For this review, take the finished solid that the model builds, in its own axes (mm). A direction names the side the tool comes from. Give positions to 0.01 mm unless a question says otherwise; leave off trailing zeros. Write each loop counter-clockwise with the first axis right and the second up, starting at its lowest first coordinate (ties: lowest second). Pieces come first, ordered by that corner, then holes.
1) We need section B-B on y = 0. Give the boundary of the cut face in (x, z).
2) For P1, Ø2, axis at x = -11.5, y = 34, coming from the +Z side; P2, Ø1.6, axis at x = -24, z = 14.5, coming from the -Y side; P3, Ø22.5, axis at y = -1.5, z = 18, coming from the -X side, all flat-tipped, find the tip position at first contact; note any pin that passes through.
3) Draft analysis for pull direction X (two halves, no side actions). For faces 4 (the face through (-11.923, 53.692, 2.348)), 5 (the face through (-23.5, 0, 23)), 6 (the face through (-24.486, -0.11, 35.764)), 7 (the face through (-1, 1, 4.762)), state which applies: pulls with the +X half, pulls with the -X half, needs draft (parallel to the pull), parting line crosses it, or undercut.
4) Wall thickness on line 1 along X through (y, z) = (-3, 9.5); line 2 along Z through (x, y) = (6.5, -30.5); line 3 along Y through (x, z) = (-25, 35.5): over which ranges is each line inside the solid? List them lowest first.
5) We need section A-A on z = 16.5. Give the boundary of the cut face in (x, y), and give its area (3 significant figures).
6) Machinability: for faces 1 (the face through (23.5, 0, 23)), 2 (the face through (-25.5, 0, 23)), 3 (the face through (25.5, 0, 23)), which of the approach directions +Z, -Z, +X, -X, +Y, -Y give a long, thin tool a straight path to every point of the face, cutting with its end or side? Answer none if there is none.
7) We need section D-D on x = 0. Give the boundary of the cut face in (y, z).
8) We need section C-C on z = 38. Give the boundary of the cut face in (x, y), and give its area (3 significant figures).
Autodesk Inventor part; units mm, degrees
ref_plane "YZ Plane" through (0, 0, 0) normal (1, 0, 0) x (0, 1, 0)
ref_plane "XZ Plane" through (0, 0, 0) normal (0, 1, 0) x (-1, 0, 0)
ref_plane "XY Plane" through (0, 0, 0) normal (0, 0, 1) x (1, 0, 0)
sketch "Sketch1" plane through (0, 0, 0) normal (0, 0, 1) x (1, 0, 0)
  circle A0 centre (0, 0) radius 55
  line L0 (23.5, -14) -> (23.5, 14)
  line L1 (-23.5, -14) -> (-23.5, 14)
  line L2 (-25.5, -14) -> (-25.5, 14)
  line L3 (25.5, -14) -> (25.5, 14)
  line L4 (25.5, 14) -> (23.5, 14)
  line L5 (23.5, -14) -> (25.5, -14)
  line L6 (-25.5, -14) -> (-23.5, -14)
  line L7 (-25.5, 14) -> (-23.5, 14)
extrude "Extrusion1" add sketch "Sketch1" along normal blind 4.7625
extrude "Extrusion2" add sketch "Sketch1" along normal blind 40.7625 contours L0 L4 L3 L5 | L6 L2 L7 L1
sketch "Sketch2" plane through (25.5, -14, 4.7625) normal (1, 0, 0) x (0, 0, -1)
  line L0 (-36, 28) -> (-36, 0)
  line L1 (-39, 7) -> (-39, 2.0417)
  arc A0 (-39, 2.0417) -> (-37.1667, 0.0487) centre (-37, 2.0417) ccw
  arc A1 (-37.1667, 0.0487) -> (-36, 0) centre (-36, 14) ccw
  line L2 (-2, 0) -> (-36, 0)
  line L3 (-2, 28) -> (-2, 0)
  line L4 (-2, 28) -> (-36, 28)
  arc A2 (-36, 28) -> (-37.1667, 27.9513) centre (-36, 14) ccw
  arc A3 (-37.1667, 27.9513) -> (-39, 25.9583) centre (-37, 25.9583) ccw
  line L5 (-39, 25.9583) -> (-39, 21)
  arc A4 (-39, 21) -> (-37, 19) centre (-37, 21) ccw
  line L6 (-37, 19) -> (-36, 19)
  arc A5 (-36, 9) -> (-36, 19) centre (-36, 14) ccw
  line L7 (-37, 9) -> (-36, 9)
  arc A6 (-37, 9) -> (-39, 7) centre (-37, 7) ccw
  circle A7 centre (-36, 25) radius 1.25
  circle A8 centre (-28.2218, 21.7782) radius 1.25
  circle A9 centre (-25, 14) radius 1.25
  circle A10 centre (-28.2218, 6.2218) radius 1.25
  circle A11 centre (-36, 3) radius 1.25
  circle A12 centre (-15, 6) radius 1.05
  circle A13 centre (-15, 22) radius 1.05
  line L8 (-8, 6) -> (-11, 6)
  arc A14 (-12, 7) -> (-11, 6) centre (-11, 7) ccw
  line L9 (-12, 7) -> (-12, 21)
  arc A15 (-11, 22) -> (-12, 21) centre (-11, 21) ccw
  line L10 (-8, 22) -> (-11, 22)
  arc A16 (-7, 21) -> (-8, 22) centre (-8, 21) ccw
  line L11 (-7, 21) -> (-7, 7)
  arc A17 (-8, 6) -> (-7, 7) centre (-8, 7) ccw
  line L12 (-18, 21) -> (-18, 7)
  arc A18 (-19, 6) -> (-18, 7) centre (-19, 7) ccw
  line L13 (-19, 6) -> (-21, 6)
  arc A19 (-22, 7) -> (-21, 6) centre (-21, 7) ccw
  line L14 (-22, 7) -> (-22, 21)
  arc A20 (-21, 22) -> (-22, 21) centre (-21, 21) ccw
  line L15 (-21, 22) -> (-19, 22)
  arc A21 (-18, 21) -> (-19, 22) centre (-19, 21) ccw
  circle A22 centre (-36, 6) radius 1
  circle A23 centre (-28, 14) radius 1
  circle A24 centre (-36, 22) radius 1
  line L16 (-36, 19) -> (-36, 9)
  point P0 (4.7625, 14)
  point P1 (-36, 14)
extrude "Extrusion3" cut sketch "Sketch2" against normal through all contours A5 L0
properties part number "Shoulder"
Results list:
1. outline: (-55, 0) - (55, 0) - (55, 4.76) - (25.5, 4.76) - (25.5, 35.76) - (23.5, 35.76) - (23.5, 4.76) - (-23.5, 4.76) - (-23.5, 35.76) - (-25.5, 35.76) - (-25.5, 4.76) - (-55, 4.76) - close
2. P1: stops at z = 4.76
2. P2: stops at y = -14
2. P3: stops at x = -25.5
3. face 4: parting line crosses it
3. face 5: undercut
3. face 6: needs draft
3. face 7: undercut
4. line 1: x = -25.5 to -23.5, 23.5 to 25.5
4. line 2: z = 0 to 4.76
4. line 3: y = -14 to 14
5. outline: (-25.5, -14) - (-23.5, -14) - (-23.5, 14) - (-25.5, 14) - close; (23.5, -14) - (25.5, -14) - (25.5, 14) - (23.5, 14) - close
5. area: 112 mm2
6. face 1: +Z, +Y, -Y
6. face 2: +Z, -X, +Y, -Y
6. face 3: +Z, +X, +Y, -Y
7. outline: (-55, 0) - (55, 0) - (55, 4.76) - (-55, 4.76) - close
8. outline: (-25.5, -14) - (-23.5, -14) - (-23.5, -4.17) - (-25.5, -4.17) - close; (-25.5, 4.17) - (-23.5, 4.17) - (-23.5, 14) - (-25.5, 14) - close; (23.5, -14) - (25.5, -14) - (25.5, -4.17) - (23.5, -4.17) - close; (23.5, 4.17) - (25.5, 4.17) - (25.5, 14) - (23.5, 14) - close
8. area: 78.7 mm2
